Check sheet for the drawn part. Datum: minimum x, y, z corner. Units: mm. A direction names the side the tool comes from. Round coordinates to 2 decimals unless told otherwise and drop trailing zeros. Write each loop counter-clockwise with the first axis right and the second up, starting at its lowest first coordinate (ties: lowest second). Pieces come first, ordered by that corner, then holes. Notation, with made-up numbers: M 35.25,63 L 52.25,63 A17 ccw 52.25,68 Z; hole C 16,38.5 d6. An arc over 180 degrees is marked long. Answer as CSV lines item,"result". Start each with the question number.
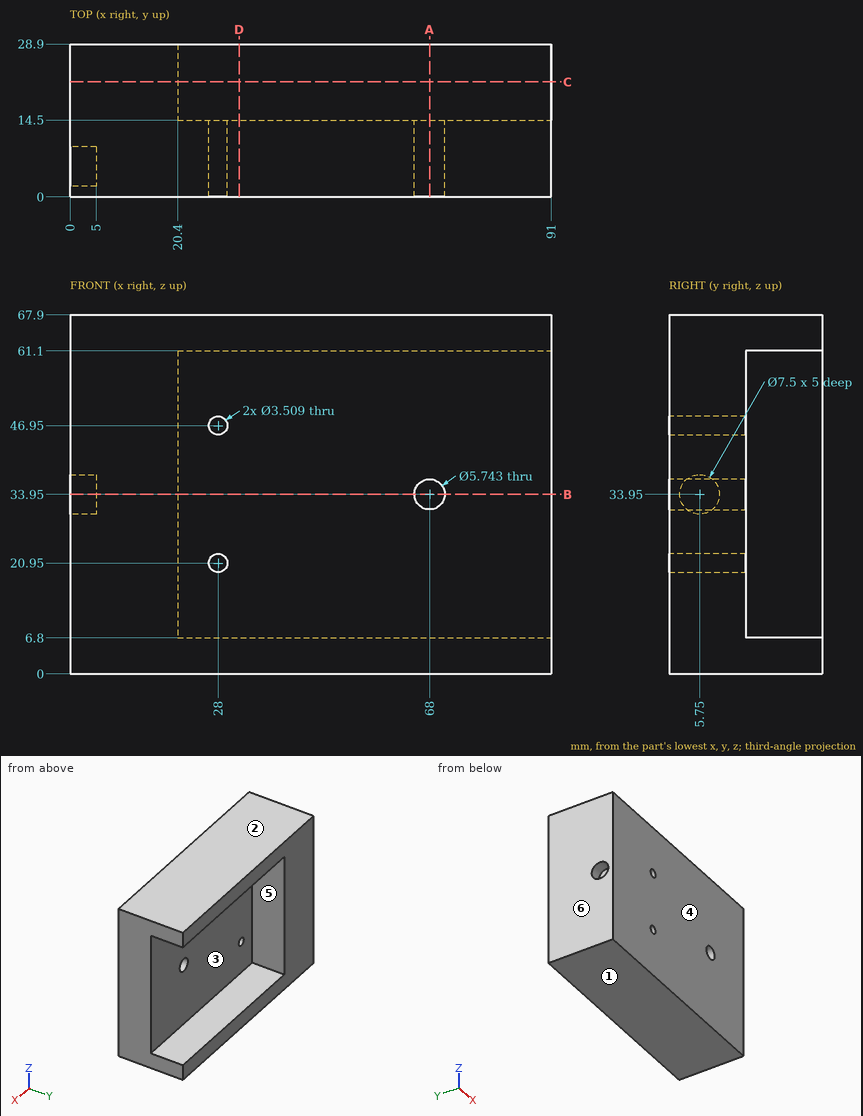
1) Section check B-B, the plane z = 33.95. Record the cut outline in (x, y).
2) Section check D-D, the plane x = 32. Record the cut outline in (y, z), plus the area to 3 significant figures.
3) Mould release check, pull along Z, two halves, no side actions. Record for the marked faces 1, 2, 3 and 4: released by +Z, released by -Z, zero draft, split by the parting line, or undercut.
4) Access from +Z, -Z, +X, -X, +Y, -Y to the whole of each face (thin tool, end or side, straight path). Record for the marked faces 5 and 6.
5) Section check C-C, the plane y = 21.75. Record the cut outline in (x, z).
6) Go/stop test with flat-tipped pins: pin 1 (2 mm diameter, centred on y = 21, z = 53.5, fed in from +X); pin 2 (2 mm diameter, centred on y = 5, z = 36, fed in from -X); pin 3 (1 mm diameter, centred on x = 42.5, z = 59.5, fed in from +Y). Record where each tip stops, or that it passes through.
7) Scan lines: line 1 (Y direction, x = 3.6, z = 33.95); line 2 (X direction, y = 5.75, z = 46.95) (1 decimal); line 3 (Z direction, x = 46, y = 19.5). Record each from-to range of solid material in increasing order. Write a range as from..to.
8) Section check A-A, the plane x = 68. Record the cut outline in (y, z).
Results:
1,outline,"M 0,0 L 65.13,0 L 65.13,14.5 L 20.4,14.5 L 20.4,28.9 L 0,28.9 L 0,9.5 L 5,9.5 L 5,2 L 0,2 Z; M 70.87,0 L 91,0 L 91,14.5 L 70.87,14.5 Z"
2,outline,"M 0,0 L 28.9,0 L 28.9,6.8 L 14.5,6.8 L 14.5,61.1 L 28.9,61.1 L 28.9,67.9 L 0,67.9 Z"
2,area,"1,180 mm^2"
3,face 1,"released by -Z"
3,face 2,"released by +Z"
3,face 3,"undercut"
3,face 4,"zero draft"
4,face 5,"+X, +Y"
4,face 6,"+Z, -Z, -X, +Y, -Y"
5,outline,"M 0,0 L 91,0 L 91,6.8 L 20.4,6.8 L 20.4,61.1 L 91,61.1 L 91,67.9 L 0,67.9 Z"
6,pin 1,"stops at x = 20.4"
6,pin 2,"stops at x = 5"
6,pin 3,"stops at y = 14.5"
7,line 1,"y = 0..2, 9.5..28.9"
7,line 2,"x = 0..26.2, 29.8..91"
7,line 3,"z = 0..6.8, 61.1..67.9"
8,outline,"M 0,0 L 28.9,0 L 28.9,6.8 L 14.5,6.8 L 14.5,31.08 L 0,31.08 Z; M 0,36.82 L 14.5,36.82 L 14.5,61.1 L 28.9,61.1 L 28.9,67.9 L 0,67.9 Z"
